```python
from build123d import *

# Parameters (mm, degrees)
SKETCH1_W           = 50
SKETCH1_H           = 14
SKETCH1_R           = 2
BOSS_EXTRUDE1_DEPTH = 5
CUT_EXTRUDE1_DEPTH  = 8
CHAMFER1_SIZE       = 2
CHAMFER1_SIZE2      = 1.154700538


with BuildPart() as part:
    # Sketch1 → Boss-Extrude1 (new body)
    with BuildSketch(Plane(origin=(0, 0, 0), x_dir=(1, 0, 0), z_dir=(0, 1, 0))):
        with Locations((0.901639344, 1.721311475)):
            Rectangle(SKETCH1_W, SKETCH1_H)
        with Locations(Location((5.901639344, 1.721311475, 0), (0, 0, 270))):
            Circle(SKETCH1_R, mode=Mode.SUBTRACT)
        with Locations(Location((-12.098360656, 1.721311475, 0), (0, 0, 270))):
            Circle(SKETCH1_R, mode=Mode.SUBTRACT)
    extrude(amount=BOSS_EXTRUDE1_DEPTH)

    # Sketch2 → Cut-Extrude1 (cut)
    with BuildSketch(Plane(origin=(25.901639344, 0, 0), x_dir=(0, 0, -1), z_dir=(1, 0, 0))):
        with BuildLine():
            Line((-0.778688525, 5), (-5.278688525, 5))
            Line((-5.278688525, 5), (-5.278688525, 0))
            Line((-5.278688525, 0), (1.721311475, 0))
            ThreePointArc((1.721311475, 0), (-0.046455478, 0.732233047), (-0.778688525, 2.5))
            Line((-0.778688525, 2.5), (-0.778688525, 5))
        make_face()
        with BuildLine():
            ThreePointArc((4.221311475, 2.5), (3.489078428, 0.732233047), (1.721311475, 0))
            Line((1.721311475, 0), (8.721311475, 0))
            Line((8.721311475, 0), (8.721311475, 5))
            Line((8.721311475, 5), (4.221311475, 5))
            Line((4.221311475, 5), (4.221311475, 2.5))
        make_face()
    extrude(amount=-CUT_EXTRUDE1_DEPTH, mode=Mode.SUBTRACT)

    # Chamfer1
    chamfer1_edges = [part.edges().sort_by_distance(p)[0] for p in [
        (5.901639344, 5, -3.721311475),
        (-12.098360656, 5, -3.721311475),
    ]]
    chamfer1_side = [part.faces().sort_by_distance(p)[0] for p in [
        (-1.439620717, 5, -1.721311475),
    ]]
    chamfer(chamfer1_edges, length=CHAMFER1_SIZE, length2=CHAMFER1_SIZE2, reference=chamfer1_side[0])


solid = part.part
```
Read the model definition and answer for the solid it produces. Units are mm, in the model's axes. A direction names the side the tool comes from. Coordinates: 2 decimals unless noted, no trailing zeros. Write each loop counter-clockwise with the first axis right and the second up, starting at its lowest first coordinate (ties: lowest second). Pieces come first, ordered by that corner, then holes. Notation, with made-up numbers: (86, -33) -> (134, -33) arc R15 cw to (134, -15) -> close; hole circle Ø5 at (61, 21). An arc over 180 degrees is marked (long way). Write item = value, one per line.
(1) Section A-A on y = 1.8 is taken. Write down the section's boundary in (x, z), plus the area to 3 significant figures.
From the geometry:
outline = (-24.1, -8.72) -> (17.9, -8.72) -> (17.9, -4.12) -> (25.9, -4.12) -> (25.9, 0.68) -> (17.9, 0.68) -> (17.9, 5.28) -> (-24.1, 5.28) -> close; hole circle Ø4 at (-12.1, -1.72); hole circle Ø4 at (5.9, -1.72)
area = 601 mm2
(2) Section C-C on x = 23 is taken. Write down the section's boundary in (y, z), plus the area to 3 significant figures.
From the geometry:
outline = (2.5, -4.22) -> (5, -4.22) -> (5, 0.78) -> (2.5, 0.78) arc R2.5 ccw to start
area = 22.3 mm2
(3) Section B-B on z = -0.75 is taken. Count the separate pieces of the cut face and the enclosed holes in it, plus the area to 3 significant figures.
From the geometry:
separate_pieces = 3
enclosed_holes = 0
area = 208 mm2
(4) Straight lines are drawn through the part: L1, parallel to X at y = 4.3, z = -3.5; L2, parallel to X at y = 3.9, z = -0.25; L3, parallel to X at y = 2.7, z = 1. For each, find the intervals that lie inside material, in ascending order. Write a range as from..to.
From the geometry:
L1 = -24.1..-14.24, -9.95..3.76, 8.05..25.9
L2 = -24.1..-13.59, -10.61..4.41, 7.39..25.9
L3 = -24.1..17.9
(5) Which of the six approach directions +Z, -Z, +X, -X, +Y, -Y give full straight-line access (tool end or side, diameter ignored) to faces 1 (the face through (22, 4, 0.779)), 2 (the face through (25.902, 2, -2))?
From the geometry:
face_1 = +Z, +X, +Y, -Y
face_2 = +Z, -Z, +X, +Y, -Y
(6) For a pull along Z with two mould halves and no side action, classify faces 3 (the face through (7.59, 1.9, -0.65)), 4 (the face through (-3, 0, -2)), 5 (the face through (22, 4, -4.221)) as +Z half, -Z half, draft (parallel to the pull), parting line (faces both ways), or undercut.
From the geometry:
face_3 = undercut
face_4 = draft
face_5 = -Z half
(7) Section D-D on z = -7.5 is taken. Write down the section's boundary in (x, y), plus the area to 3 significant figures.
From the geometry:
outline = (-24.1, 0) -> (17.9, 0) -> (17.9, 5) -> (-24.1, 5) -> close
area = 210 mm2
(8) Given pin 1 Ø6.5 at (x, z) = (5.9, -1.72) entering from +Y; pin 2 Ø3 at (x, y) = (21.5, 4) entering from +Z; pin 3 Ø2 at (x, y) = (22.5, 4) entering from -Z, each flat-ended and moving along its own axis, determine where each tip first touches the part or whether it passes through.
From the geometry:
pin_1 = 4.57
pin_2 = 0.78
pin_3 = -4.22
